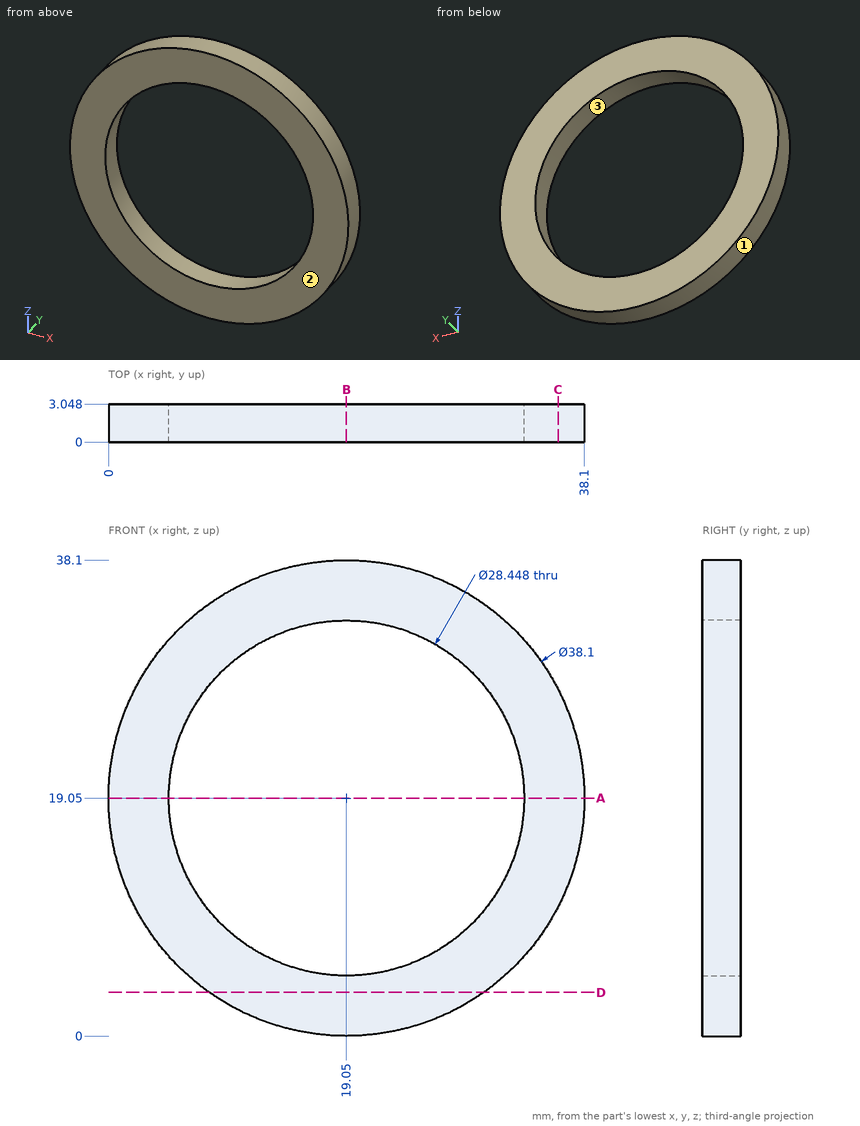
The figure shows three views and two pictorial views of one solid part (mm, origin at its lowest corner). Answer the questions. Round coordinates to 2 decimals unless told otherwise and drop trailing zeros. Write each loop counter-clockwise with the first axis right and the second up, starting at its lowest first coordinate (ties: lowest second). Pieces come first, ordered by that corner, then holes. Notation, with made-up numbers: M 52.5,81.5 L 56.5,81.5 A10 cw 56.5,86.5 Z; hole C 43,79.5 d7. An arc over 180 degrees is marked long. Use a Markdown table: item, result.
1) The part is cut by section D-D on z = 3.5. Give the vertices of the cut face in (x, y), plus the area to 3 significant figures.
Taken from the geometry:
| item | result |
|---|---|
| outline | M 8.05,0 L 30.05,0 L 30.05,3.05 L 8.05,3.05 Z |
| area | 67.1 mm2 |
2) The part is cut by section A-A on z = 19.05. Give the vertices of the cut face in (x, y).
Taken from the geometry:
| item | result |
|---|---|
| outline | M 0,0 L 4.83,0 L 4.83,3.05 L 0,3.05 Z; M 33.27,0 L 38.1,0 L 38.1,3.05 L 33.27,3.05 Z |
3) A flat-ended cylindrical pin translates along its axis: pin 1 (1 mm diameter, centred on x = 24, y = 2, fed in from +Z). Find the tip coordinate at first contact, or state that the pin passes through.
Taken from the geometry:
| item | result |
|---|---|
| pin 1 | stops at z = 37.57 |
4) Determine the mould class of the marked faces 1, 2 and 3 for opening direction X: pulls with the +X half, pulls with the -X half, needs draft (parallel to the pull), parting line crosses it, or undercut.
Taken from the geometry:
| item | result |
|---|---|
| face 1 | parting line crosses it |
| face 2 | needs draft |
| face 3 | undercut |
5) The part is cut by section C-C on x = 36. Give the vertices of the cut face in (y, z), plus the area to 3 significant figures.
Taken from the geometry:
| item | result |
|---|---|
| outline | M 0,10.36 L 3.05,10.36 L 3.05,27.74 L 0,27.74 Z |
| area | 53.0 mm2 |
6) The part is cut by section B-B on x = 19.05. Give the vertices of the cut face in (y, z), plus the area to 3 significant figures.
Taken from the geometry:
| item | result |
|---|---|
| outline | M 0,0 L 3.05,0 L 3.05,4.83 L 0,4.83 Z; M 0,33.27 L 3.05,33.27 L 3.05,38.1 L 0,38.1 Z |
| area | 29.4 mm2 |
7) Consider line 1 (X direction, y = 1.5, z = 19.05); line 2 (Z direction, x = 16.5, y = 0.9); line 3 (Z direction, x = 23, y = 1.05). Determine where each line is inside the solid, lowest interval first. Write a range as [from, to].
Taken from the geometry:
| item | result |
|---|---|
| line 1 | x = [0, 4.83], [33.27, 38.1] |
| line 2 | z = [0.17, 5.06], [33.04, 37.93] |
| line 3 | z = [0.41, 5.39], [32.71, 37.69] |
